For this review, use the dimensioned drawing (mm, ordinates from the lowest corner) and the shaded views. A direction names the side the tool comes from. Give positions to 0.01 mm unless a question says otherwise; leave off trailing zeros. Write each loop counter-clockwise with the first axis right and the second up, starting at its lowest first coordinate (ties: lowest second). Pieces come first, ordered by that corner, then holes.
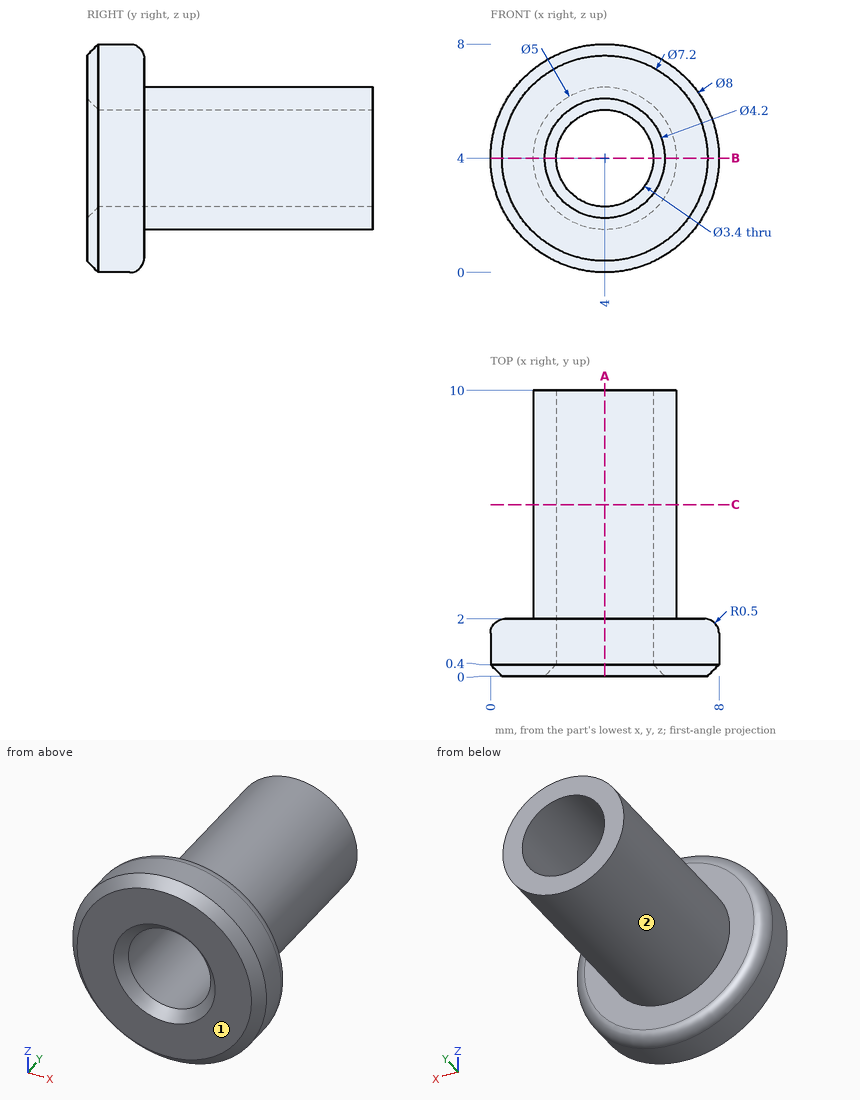
(1) Clearance check with flat-ended pins moving along their axes: pin 1 Ø2 at (x, z) = (7, 6) entering from +Y; pin 2 Ø1.5 at (x, y) = (6, 1.5) entering from -Z; pin 3 Ø1.5 at (x, y) = (1, 3) entering from -Z. State where each tip first meets the part, or that it passes through.
(2) Tool access review of the marked faces 1 and 2: name each direction out of +Z, -Z, +X, -X, +Y, -Y from which nothing blocks a thin tool from reaching the whole face with its end or side.
(3) We need section A-A (x = 4). Write out the cut boundary in (y, z).
(4) We need section B-B (z = 4). Write out the cut boundary in (x, y).
(5) For L1, parallel to X at y = 3.5, z = 4; L2, parallel to Y at x = 2, z = 1.5; L3, parallel to Z at x = 2.5, y = 0.75, list the stretches that pass through material, from the lowest coordinate up.
(6) We need section C-C (y = 6). Write out the cut boundary in (x, z).
The answers:
1. pin 1: stops at y = 2
1. pin 2: stops at z = 0.2
1. pin 3: stops at z = 2.91
2. face 1: +Z, -Z, +X, -X, -Y
2. face 2: +Y
3. outline: (0, 0.4) - (0.4, 0) - (1.5, 0) arc R0.5 ccw to (2, 0.5) - (2, 1.5) - (10, 1.5) - (10, 2.3) - (0.4, 2.3) - (0, 1.9) - close; (0, 6.1) - (0.4, 5.7) - (10, 5.7) - (10, 6.5) - (2, 6.5) - (2, 7.5) arc R0.5 ccw to (1.5, 8) - (0.4, 8) - (0, 7.6) - close
4. outline: (0, 0.4) - (0.4, 0) - (1.9, 0) - (2.3, 0.4) - (2.3, 10) - (1.5, 10) - (1.5, 2) - (0.5, 2) arc R0.5 ccw to (0, 1.5) - close; (5.7, 0.4) - (6.1, 0) - (7.6, 0) - (8, 0.4) - (8, 1.5) arc R0.5 ccw to (7.5, 2) - (6.5, 2) - (6.5, 10) - (5.7, 10) - close
5. L1: x = 1.5 to 2.3, 5.7 to 6.5
5. L2: y = 0 to 2
5. L3: z = 0.29 to 3.2, 4.8 to 7.71
6. outline: circle Ø5 at (4, 4); hole circle Ø3.4 at (4, 4)
